Geometry check sheet. Reference: the model listing, model coordinates, mm. Give positions to 0.01 mm unless a question says otherwise; leave off trailing zeros. Loops run counter-clockwise (first coordinate to the right, second up) from the corner with the lowest first, then second, coordinate; pieces in that order, holes last. Notation, with made-up numbers: (55.5, -17) - (101.5, -17) arc R22 ccw to (101.5, 8) - close; hole circle Ø6 at (-21.75, 18). An arc over 180 degrees is marked (long way). Write item = value, one per line. Start each with the question number.
from build123d import *

# Parameters (mm, degrees)
SKETCH1_W           = 2438.4
SKETCH1_H           = 1219.2
BOSS_EXTRUDE1_DEPTH = 19.05
SKETCH2_W           = 869.95
SKETCH2_H           = 534.9875
CUT_EXTRUDE1_DEPTH  = 20.05
SKETCH3_W           = 508
SKETCH3_H           = 685.8
CUT_EXTRUDE2_DEPTH  = 20.05
SKETCH4_W           = 676.20134
SKETCH4_H           = 863.85146
CUT_EXTRUDE3_DEPTH  = 20.05
SKETCH5_W           = 846.4296
SKETCH5_H           = 206.375
CUT_EXTRUDE4_DEPTH  = 20.05
CUT_EXTRUDE6_DEPTH  = 20.05
CUT_EXTRUDE7_DEPTH  = 846.4296


with BuildPart() as part:
    # Sketch1 → Boss-Extrude1 (new body)
    with BuildSketch(Plane(origin=(0, 0, 0), x_dir=(1, 0, 0), z_dir=(0, 1, 0))):
        with Locations((1219.2, 609.6)):
            Rectangle(SKETCH1_W, SKETCH1_H)
    extrude(amount=-BOSS_EXTRUDE1_DEPTH)

    # Sketch2 → Cut-Extrude1 (cut, through all)
    with BuildSketch(Plane(origin=(0, 0, 0), x_dir=(1, 0, 0), z_dir=(0, 1, 0))):
        with Locations((1917.065, 318.29375)):
            Rectangle(SKETCH2_W, SKETCH2_H)
    extrude(amount=-CUT_EXTRUDE1_DEPTH, mode=Mode.SUBTRACT)

    # Sketch3 → Cut-Extrude2 (cut, through all)
    with BuildSketch(Plane(origin=(0, 0, 0), x_dir=(1, 0, 0), z_dir=(0, 1, 0))):
        with Locations((1046.1625, 342.9)):
            Rectangle(SKETCH3_W, SKETCH3_H)
    extrude(amount=-CUT_EXTRUDE2_DEPTH, mode=Mode.SUBTRACT)

    # Sketch4 → Cut-Extrude3 (cut, through all)
    with BuildSketch(Plane(origin=(0, 0, 0), x_dir=(1, 0, 0), z_dir=(0, 1, 0))):
        with Locations((1914.52627, 1260.98427)):
            Rectangle(SKETCH4_W, SKETCH4_H)
    extrude(amount=-CUT_EXTRUDE3_DEPTH, mode=Mode.SUBTRACT)

    # Sketch5 → Cut-Extrude4 (cut, through all)
    with BuildSketch(Plane(origin=(0, 0, 0), x_dir=(1, 0, 0), z_dir=(0, 1, 0))):
        with Locations((722.3252, 1116.0125)):
            Rectangle(SKETCH5_W, SKETCH5_H)
    extrude(amount=-CUT_EXTRUDE4_DEPTH, mode=Mode.SUBTRACT)

    # Sketch8 → Cut-Extrude6 (cut, through all)
    with BuildSketch(Plane(origin=(0, 0, 0), x_dir=(1, 0, 0), z_dir=(0, 1, 0))):
        Polygon((294.0685, 704.85), (275.0185, 685.8), (275.0185, 450.85), (294.0685, 431.8), (465.5185, 431.8), (484.5685, 450.85), (484.5685, 685.8), (465.5185, 704.85), align=None)
    extrude(amount=-CUT_EXTRUDE6_DEPTH, mode=Mode.SUBTRACT)

    # Sketch9 → Cut-Extrude7 (cut)
    with BuildSketch(Plane.ZY.offset(-299.1104)):
        with BuildLine():
            Line((-1009.601754844, 0), (-1219.2, 0))
            Line((-1219.2, 0), (-1219.2, -19.05))
            Line((-1219.2, -19.05), (-1005.293201675, -19.05))
            ThreePointArc((-1005.293201675, -19.05), (-1007.340207177, -9.500738417), (-1009.601754844, 0))
        make_face()
    extrude(amount=-CUT_EXTRUDE7_DEPTH, mode=Mode.SUBTRACT)


solid = part.part
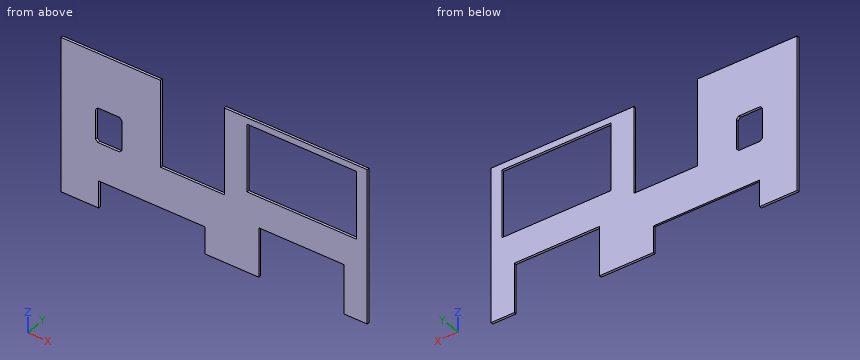
1) Cross-section at B-B on z = -1055.5. Enter the section's corners in (x, y).
2) Cross-section at A-A on x = 1713.5. Enter the section's corners in (y, z).
3) Material ranges on line 1 along X through (y, z) = (-3.25, -469.5); line 2 along X through (y, z) = (-0.75, -356); line 3 along X through (y, z) = (-9.5, -1125.5), recorded low to high.
4) Cross-section at C-C on z = -859. Enter the section's corners in (x, y), and give its area (3 significant figures).
5) Cross-section at D-D on y = -6. Enter the section's corners in (x, z).
6) Gauge pin test, flat ends, axial feed: P1, Ø9.5, axis at x = 1088, y = -13, coming from the +Z side; P2, Ø5.5, axis at x = 349, y = -10, coming from the -Z side. Record the tip position at first contact, or that the pin passes through.
Checked values:
q1.outline = (0, -19.05) - (299.11, -19.05) - (299.11, 0) - (0, 0) - close; (1145.54, -19.05) - (1576.43, -19.05) - (1576.43, 0) - (1145.54, 0) - close; (2252.63, -19.05) - (2438.4, -19.05) - (2438.4, 0) - (2252.63, 0) - close
q2.outline = (-19.05, -829.06) - (0, -829.06) - (0, -585.79) - (-19.05, -585.79) - close; (-19.05, -50.8) - (0, -50.8) - (0, 0) - (-19.05, 0) - close
q3.line_1 = 0 to 275.02, 484.57 to 792.16, 1300.16 to 1482.09, 2352.04 to 2438.4
q3.line_2 = 0 to 792.16, 1300.16 to 1482.09, 2352.04 to 2438.4
q3.line_3 = 0 to 299.11, 1145.54 to 1576.43, 2252.63 to 2438.4
q4.outline = (0, -19.05) - (1576.43, -19.05) - (1576.43, 0) - (0, 0) - close; (2252.63, -19.05) - (2438.4, -19.05) - (2438.4, 0) - (2252.63, 0) - close
q4.area = 33,600 mm²
q5.outline = (0, -1219.2) - (299.11, -1219.2) - (299.11, -1008.15) - (1145.54, -1008.15) - (1145.54, -1219.2) - (1576.43, -1219.2) - (1576.43, -829.06) - (2252.63, -829.06) - (2252.63, -1219.2) - (2438.4, -1219.2) - (2438.4, 0) - (1300.16, 0) - (1300.16, -685.8) - (792.16, -685.8) - (792.16, 0) - (0, 0) - close; hole (275.02, -685.8) - (294.07, -704.85) - (465.52, -704.85) - (484.57, -685.8) - (484.57, -450.85) - (465.52, -431.8) - (294.07, -431.8) - (275.02, -450.85) - close; hole (1482.09, -585.79) - (2352.04, -585.79) - (2352.04, -50.8) - (1482.09, -50.8) - close
q6.P1 = -685.8
q6.P2 = -1007.86
